```python
from build123d import *

# Parameters (mm, degrees)
SKETCH2_W           = 69.85
SKETCH2_H           = 7.62
BOSS_EXTRUDE1_DEPTH = 2.54
FILLET1_RADIUS      = 3.81
FILLET1_LENGTH      = 2.54
FILLET2_RADIUS      = 3.81
FILLET2_LENGTH      = 2.54
SKETCH3_R           = 1.27
BOSS_EXTRUDE2_DEPTH = 2.54


with BuildPart() as part:
    # Sketch2 → Boss-Extrude1 (new body)
    with BuildSketch(Plane(origin=(0, 0, 0), x_dir=(1, 0, 0), z_dir=(0, 1, 0))):
        Rectangle(SKETCH2_W, SKETCH2_H)
    extrude(amount=BOSS_EXTRUDE1_DEPTH)

    # Fillet1: full round fillet: the end face becomes a half cylinder, R = half its width
    fillet1_face = Plane((34.925, 1.27, 0), x_dir=(0, 1, 0), z_dir=(1, 0, 0))  # on the end face: x along it, z out of the body
    fillet1_slab = fillet1_face.offset(-FILLET1_RADIUS / 2) * Box(FILLET1_LENGTH, 2 * FILLET1_RADIUS, FILLET1_RADIUS, mode=Mode.PRIVATE)  # the body's end, R deep
    fillet1_round = Plane((31.115, 1.27, 0), x_dir=(1, 0, 0), z_dir=(0, 1, 0)) * Cylinder(FILLET1_RADIUS, FILLET1_LENGTH, mode=Mode.PRIVATE)  # its axis R under the face
    add(fillet1_slab - fillet1_round, mode=Mode.SUBTRACT)

    # Fillet2: full round fillet: the end face becomes a half cylinder, R = half its width
    fillet2_face = Plane((-34.925, 1.27, 0), x_dir=(0, -1, 0), z_dir=(-1, 0, 0))  # on the end face: x along it, z out of the body
    fillet2_slab = fillet2_face.offset(-FILLET2_RADIUS / 2) * Box(FILLET2_LENGTH, 2 * FILLET2_RADIUS, FILLET2_RADIUS, mode=Mode.PRIVATE)  # the body's end, R deep
    fillet2_round = Plane((-31.115, 1.27, 0), x_dir=(-1, 0, 0), z_dir=(0, -1, 0)) * Cylinder(FILLET2_RADIUS, FILLET2_LENGTH, mode=Mode.PRIVATE)  # its axis R under the face
    add(fillet2_slab - fillet2_round, mode=Mode.SUBTRACT)

    # Sketch3 → Boss-Extrude2 (add)
    with BuildSketch(Plane(origin=(0, 2.54, 0), x_dir=(1, 0, 0), z_dir=(0, 1, 0))):
        with Locations(Location((-31.227747573, 0, 0), (0, 0, 270))):
            Circle(SKETCH3_R)
    extrude(amount=BOSS_EXTRUDE2_DEPTH)


solid = part.part
```
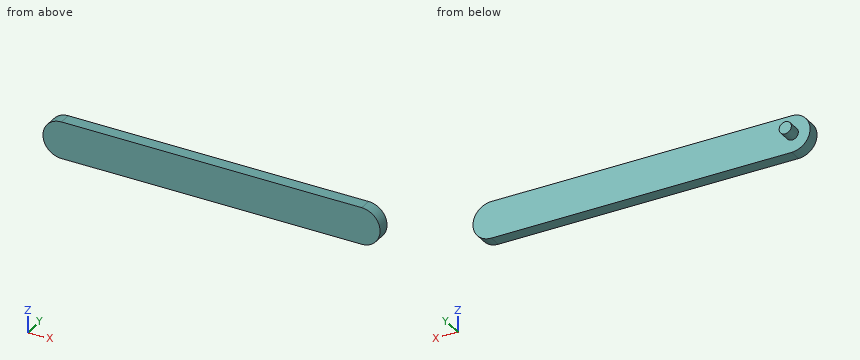
Could you check a few things on this model? Use its own coordinates, in mm. Round coordinates to 2 decimals unless told otherwise and drop trailing zeros. Loops run counter-clockwise (first coordinate to the right, second up) from the corner with the lowest first, then second, coordinate; pieces in that order, holes last. Notation, with made-up numbers: M 64,-29.5 L 119,-29.5 A23 cw 119,1.5 Z; hole C -35,-5 d4. An arc over 180 degrees is marked long. Answer as CSV lines item,"result".
1) If I drill on probe 1 along Y at (x, z) = (-23, -0.75); probe 2 along X at (y, z) = (2.2, 1.5); probe 3 along X at (y, z) = (0.25, -1), over which ranges is the centre line in solid material (lowest first)?
From the geometry:
probe 1,"0 to 2.54"
probe 2,"-34.62 to 34.62"
probe 3,"-34.79 to 34.79"
2) Imagine slicing it at C-C on x = -1. List the corners of the cut face in (y, z) for me.
From the geometry:
outline,"M 0,-3.81 L 2.54,-3.81 L 2.54,3.81 L 0,3.81 Z"
3) Imagine slicing it at A-A on z = 0. List the corners of the cut face in (x, y) for me (3 decimals).
From the geometry:
outline,"M -34.925,0 L 34.925,0 L 34.925,2.54 L -29.958,2.54 L -29.958,5.08 L -32.498,5.08 L -32.498,2.54 L -34.925,2.54 Z"
4) Imagine slicing it at B-B on y = 1.7. List the corners of the cut face in (x, z) for me (3 decimals), and give its area (3 significant figures).
From the geometry:
outline,"M -31.115,-3.81 L 31.115,-3.81 A3.81 ccw 31.115,3.81 L -31.115,3.81 A3.81 ccw Z"
area,"520 mm^2"
